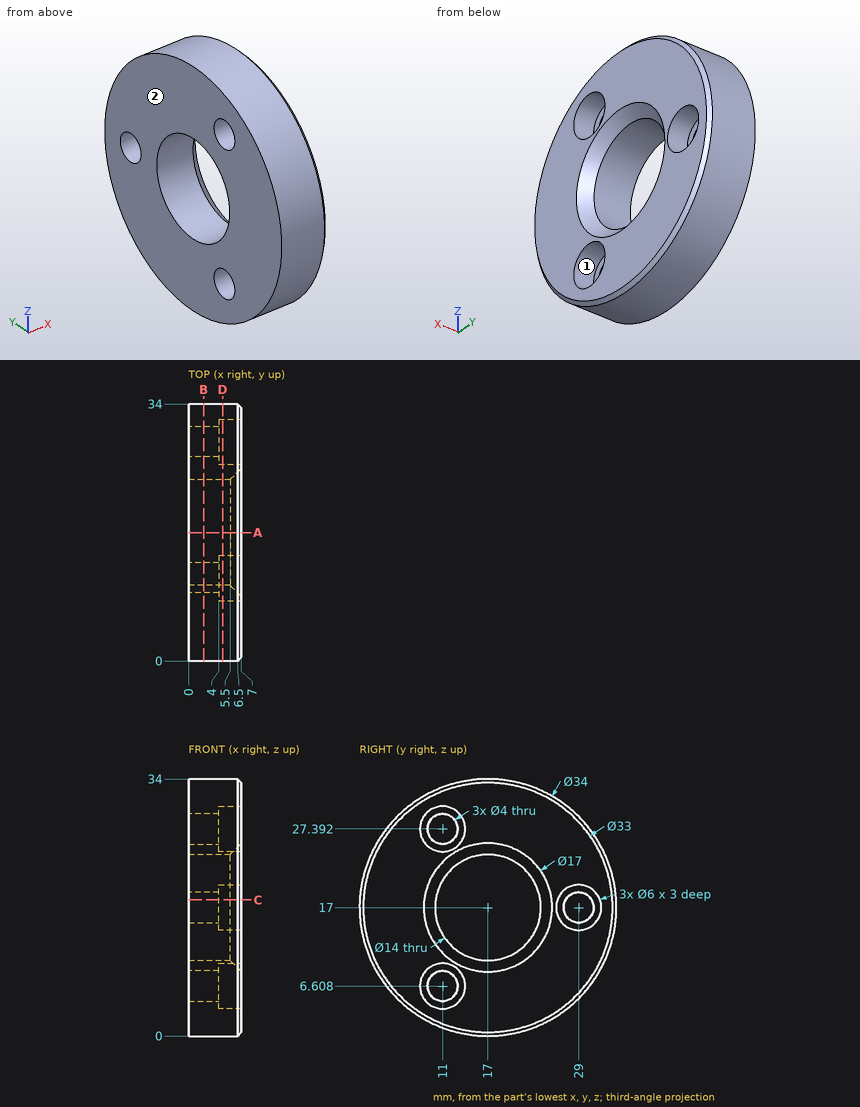
Check sheet for the drawn part. Datum: minimum x, y, z corner. Units: mm. A direction names the side the tool comes from. Coordinates: 2 decimals unless noted, no trailing zeros. Write each loop counter-clockwise with the first axis right and the second up, starting at its lowest first coordinate (ties: lowest second). Pieces come first, ordered by that corner, then holes. Notation, with made-up numbers: (35.5, 57.5) - (83.5, 57.5) arc R20 cw to (83.5, 75.5) - close; hole circle Ø7 at (57.25, 64.25). An arc over 180 degrees is marked (long way). Answer as a JSON object with one key per item and string values.
(1) Cross-section at C-C on z = 18. Give the number of separate pieces and of enclosed holes in the cut face, plus the area to 3 significant figures.
Report:
{"separate pieces": "3", "enclosed holes": "0", "area": "107 mm^2"}
(2) Cross-section at B-B on x = 2. Record the cut outline in (y, z), plus the area to 3 significant figures.
Report:
{"outline": "circle Ø34 at (17, 17); hole circle Ø4 at (11, 6.61); hole circle Ø4 at (11, 27.39); hole circle Ø14 at (17, 17); hole circle Ø4 at (29, 17)", "area": "716 mm^2"}
(3) Cross-section at D-D on x = 4.5. Record the cut outline in (y, z), plus the area to 3 significant figures.
Report:
{"outline": "circle Ø34 at (17, 17); hole circle Ø6 at (11, 6.61); hole circle Ø6 at (11, 27.39); hole circle Ø14 at (17, 17); hole circle Ø6 at (29, 17)", "area": "669 mm^2"}
(4) Thickness scan on line 1 along Y through (x, z) = (5.5, 17); line 2 along Y through (x, z) = (5.9, 17); line 3 along Z through (x, y) = (0.95, 11) (1 decimal). Record the ranges inside material, lowest first.
Report:
{"line 1": "0 to 10, 24 to 26, 32 to 34", "line 2": "0 to 9.6, 24.4 to 26, 32 to 34", "line 3": "1.1 to 4.6, 8.6 to 13.4, 20.6 to 25.4, 29.4 to 32.9"}
(5) Cross-section at A-A on y = 17. Record the cut outline in (x, z).
Report:
{"outline": "(0, 0) - (6.5, 0) - (7, 0.5) - (7, 8.5) - (5.5, 10) - (0, 10) - close; (0, 24) - (5.5, 24) - (7, 25.5) - (7, 33.5) - (6.5, 34) - (0, 34) - close"}
(6) Tool access check on the marked faces 1 and 2. Record the directions out of +Z, -Z, +X, -X, +Y, -Y that give a thin tool (end or side, any length) a straight path to the whole face; none if there is none.
Report:
{"face 1": "+X", "face 2": "+Z, -Z, -X, +Y, -Y"}
(7) Gauge pin test, flat ends, axial feed: pin 1 Ø3 at (y, z) = (9.5, 26.5) entering from +X; pin 2 Ø4 at (x, z) = (1, 11) entering from +Y; pin 3 Ø1 at (x, y) = (4.5, 6.5) entering from +Z; pin 4 Ø3.5 at (y, z) = (29, 17) entering from -X. Record the tip position at first contact, or that the pin passes through.
Report:
{"pin 1": "x = 7", "pin 2": "y = 33.52", "pin 3": "z = 30.75", "pin 4": "through"}
